from build123d import *

# Parameters (mm, degrees)
F0_R      = 2.4
F1_DEPTH  = 10.36
F0_R_2    = 4.5
F1_FACE_R = 2.4
F2_DEPTH  = 5
F3_R      = 3
F4_DEPTH  = 3


with BuildPart() as f1:
    # F0 (on Top) → F1 (new body)
    with BuildSketch(Plane.XY):
        Circle(F0_R)
    extrude(amount=F1_DEPTH)

    # F0 (on Top) + F1_face (on face) → F2 (join)
    with BuildSketch(Plane.XY):
        Circle(F0_R_2)
        Circle(F0_R, mode=Mode.SUBTRACT)
    with BuildSketch(Plane(origin=(0, 0, 0), x_dir=(1, 0, 0), z_dir=(0, 0, -1))):
        Circle(F1_FACE_R)
    extrude(amount=-F2_DEPTH, dir=(0, 0, 1))

    # F3 (on face) → F4 (cut)
    with BuildSketch(Plane(origin=(0, 0, -5), x_dir=(1, 0, 0), z_dir=(0, 0, -1))):
        Circle(F3_R)
    extrude(amount=-F4_DEPTH, mode=Mode.SUBTRACT)


solid = f1.part
Geometry: final body of the model. Coordinates: model frame, mm. A direction names the side the tool comes from. Give positions to 0.01 mm unless a question says otherwise; leave off trailing zeros. Order: outer loops, then holes, each group sorted by start corner. A loop starts at its lowest first (then second) coordinate and runs counter-clockwise, first axis right, second up. Notation, with made-up numbers: (-3.75, 31.5) -> (36.25, 31.5) arc R20 ccw to (36.25, 44.5) -> close; hole circle Ø3 at (23.5, 67). An arc over 180 degrees is marked (long way). Put each result on its own line as item: value.
Q1. Reachability of faces 1 (the face through (0, 0, -2)), 2 (the face through (1, -3, -5)) from +Z, -Z, +X, -X, +Y, -Y: full face, straight path, thin tool, end or side. Return the list, or none.
Here are the results:
face 1: -Z
face 2: -Z, +X, -X, +Y, -Y
Q2. Section D-D, the plane z = 0.75. Return loops of the section in (x, y).
Here are the results:
outline: circle Ø4.8 at (0, 0)
Q3. Material intervals for L1, parallel to Y at x = 0, z = -3.2; L2, parallel to Z at x = 1.5, y = 3.5; L3, parallel to Y at x = -0.75, z = -3, sorted ascending.
Here are the results:
L1: y = -4.5 to -3, 3 to 4.5
L2: z = -5 to 0
L3: y = -4.44 to -2.9, 2.9 to 4.44
Q4. Draft query along Y for faces 3 (the face through (-3, 0, -4)), 4 (the face through (1.29, 2.024, 5.107)), 5 (the face through (2, -2, 0)). Return one class per face: released by +Y, released by -Y, zero draft, split by the parting line, or undercut.
Here are the results:
face 3: undercut
face 4: split by the parting line
face 5: zero draft
Q5. Section A-A, the plane x = 0. Return loops of the section in (y, z).
Here are the results:
outline: (-4.5, -5) -> (-3, -5) -> (-3, -2) -> (3, -2) -> (3, -5) -> (4.5, -5) -> (4.5, 0) -> (2.4, 0) -> (2.4, 10.36) -> (-2.4, 10.36) -> (-2.4, 0) -> (-4.5, 0) -> close
Q6. Pin query (flat end, axial travel): pin 1 (1.5 mm diameter, centred on x = -2, z = 6.5, fed in from +Y); pin 2 (3 mm diameter, centred on x = 3.5, z = -0.5, fed in from +Y); pin 3 (1.8 mm diameter, centred on x = 0, y = -1, fed in from -Z). Return the tip coordinate at first contact, or that it passes through.
Here are the results:
pin 1: stops at y = 2.05
pin 2: stops at y = 4.03
pin 3: stops at z = -2
Q7. Section C-C, the plane y = -1. Return loops of the section in (x, z).
Here are the results:
outline: (-4.39, -5) -> (-2.83, -5) -> (-2.83, -2) -> (2.83, -2) -> (2.83, -5) -> (4.39, -5) -> (4.39, 0) -> (2.18, 0) -> (2.18, 10.36) -> (-2.18, 10.36) -> (-2.18, 0) -> (-4.39, 0) -> close
Q8. Section B-B, the plane z = -3. Return loops of the section in (x, y), then the cut area to 3 significant figures.
Here are the results:
outline: circle Ø9 at (0, 0); hole circle Ø6 at (0, 0)
area: 35.3 mm^2
